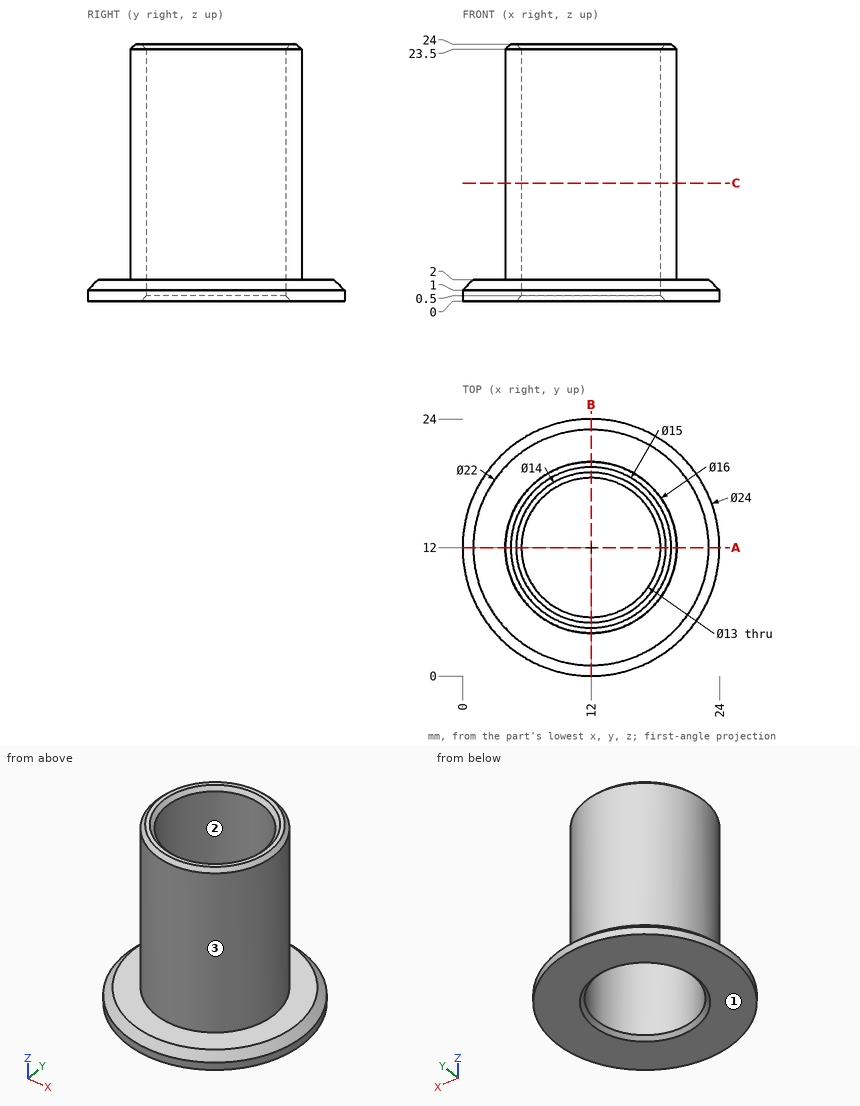
Input: dimensioned drawing with shaded views. Units: mm. Origin: part minimum x, y, z. Give positions to 0.01 mm unless a question says otherwise; leave off trailing zeros. Order: outer loops, then holes, each group sorted by start corner. A loop starts at its lowest first (then second) coordinate and runs counter-clockwise, first axis right, second up. Notation, with made-up numbers: (5.5, 24.5) -> (10.5, 24.5) arc R12 cw to (10.5, 39.5) -> close; hole circle Ø6 at (76, 47). An arc over 180 degrees is marked (long way). Use one line per item in the form item = value.
1) First-contact query: pin 1 Ø4 at (y, z) = (15, 12) entering from +X; pin 2 Ø3 at (y, z) = (13.5, 20.5) entering from -X; pin 3 Ø10 at (y, z) = (12.5, 15) entering from +X. Flat tips, straight axial feed; report the tip coordinate or a pass-through.
Response values:
pin_1 = 19.94
pin_2 = 4
pin_3 = 20
2) Mould query, pull axis Y, two halves, no side actions, for the marked faces 1, 2 and 3. Classes: pulls with the +Y half, pulls with the -Y half, needs draft (parallel to the pull), parting line crosses it, or undercut.
Response values:
face_1 = needs draft
face_2 = undercut
face_3 = parting line crosses it
3) Section A-A, the plane y = 12. Return loops of the section in (x, z).
Response values:
outline = (0, 0) -> (5, 0) -> (5.5, 0.5) -> (5.5, 23.5) -> (5, 24) -> (4.5, 24) -> (4, 23.5) -> (4, 2) -> (1, 2) -> (0, 1) -> close; (18.5, 0.5) -> (19, 0) -> (24, 0) -> (24, 1) -> (23, 2) -> (20, 2) -> (20, 23.5) -> (19.5, 24) -> (19, 24) -> (18.5, 23.5) -> close
4) Section C-C, the plane z = 11. Return loops of the section in (x, y).
Response values:
outline = circle Ø16 at (12, 12); hole circle Ø13 at (12, 12)
5) Line query: probe 1 along Y at (x, z) = (12, 16.5); probe 2 along Y at (x, z) = (10, 9); probe 3 along Z at (x, y) = (7, 5.25). Output: solid intervals per line, ascending.
Response values:
probe_1 = 4 to 5.5, 18.5 to 20
probe_2 = 4.25 to 5.82, 18.18 to 19.75
probe_3 = 0 to 2
